Autodesk Inventor part; units mm, degrees
ref_plane "YZ Plane" through (0, 0, 0) normal (1, 0, 0) x (0, 1, 0)
ref_plane "XZ Plane" through (0, 0, 0) normal (0, 1, 0) x (-1, 0, 0)
ref_plane "XY Plane" through (0, 0, 0) normal (0, 0, 1) x (1, 0, 0)
sketch "Sketch1" plane through (0, 0, 0) normal (0, 1, 0) x (-1, 0, 0)
  circle A0 centre (0, 0) radius 4
  dimension "d0" = 8
extrude "Extrusion1" add sketch "Sketch1" along normal blind 36
sketch "Sketch2" plane through (0, 36, 0) normal (0, 1, 0) x (1, 0, 0)
  line L0 (0, -2) -> (2.3553, -2)
  line L1 (-0.9798, -0.8) -> (0.9798, -0.8)
  arc A0 (0.9798, -0.8) -> (-0.9798, -0.8) centre (0, -0.3) ccw
  circle A1 centre (0, 0) radius 4
  line L2 (5.6, 0) -> (-5.6, 0)
  dimension "d4" = 1.2
  dimension "d6" = 1.1
  dimension "d7" = 0.3
extrude "Extrusion2" add sketch "Sketch2" along normal blind 11.25 contours A0 L2 L1 | A0 L2
sketch "Sketch3" plane through (0, 0, 0) normal (0, -1, 0) x (1, 0, 0)
  line L0 (-0.9798, 0.8) -> (0.9798, 0.8)
  arc A0 (-0.9798, 0.8) -> (0.9798, 0.8) centre (0, 0.3) ccw
  point P0 (0, 0)
  point P1 (0, 0)
  point P2 (0, 0.8)
  dimension "d12" = 1.9596
  dimension "d16" = 1.1
  dimension "d17" = 0.3
extrude "Extrusion3" add sketch "Sketch3" along normal blind 9
sketch "Sketch5" plane through (0, 0, 0) normal (0, -1, 0) x (1, 0, 0)
  circle A0 centre (0, 0) radius 5.5
  dimension "d29" = 11
extrude "Extrusion5" add sketch "Sketch5" against normal blind 2
chamfer "Chamfer3" distance 0.5 angle 45 2 edges at (-5.5, 0, 0) (-5.5, 2, 0)
equation "\"d4\" = d3"
properties part number "axle-skibidi"
Here's how the part is built. I have some questions about the finished solid (model axes, mm). A direction names the side the tool comes from. Round coordinates to 2 decimals unless told otherwise and drop trailing zeros. Write each loop counter-clockwise with the first axis right and the second up, starting at its lowest first coordinate (ties: lowest second). Pieces come first, ordered by that corner, then holes. Notation, with made-up numbers: M 62.25,16 L 84.25,16 A27 ccw 84.25,45 Z; hole C -1.5,26.25 d8. An arc over 180 degrees is marked long. Answer as CSV lines item,"result". Start each with the question number.
1. I need wall thicknesses on probe 1 along X at (y, z) = (1, 0.25); probe 2 along X at (y, z) = (-4.5, 0.25); probe 3 along Y at (x, z) = (0.75, 2). Which ranges of each line are inside material? Lowest first, please.
2. Suppose I cut it at D-D on y = -0.5. Write out the boundary of the cut face in (x, z).
3. On a 3-axis mill with a long thin cutter (end or side, diameter ignored), from which of +Z, -Z, +X, -X, +Y, -Y can I reach the whole of each face in a straight line? I mean faces 1 (the flat face through (0, -4, 0.8)), 2 (the cylindrical face through (0, 41.5, -0.8)), 3 (the flat face through (0, 42, 0.8)), 4 (the flat face through (0, 47.25, 0)), 5 (the cylindrical face through (0, -4.4, -0.8)). Say none if no direction works.
4. I'm going to push flat-ended pins straight in: pin 1 Ø4 at (x, y) = (-2, 23.5) entering from +Z; pin 2 Ø3 at (x, y) = (4, 30) entering from +Z; pin 3 Ø1.6 at (x, y) = (0.5, 44) entering from +Z. Where does each tip first touch, or does it pass through?
5. Suppose I cut it at A-A on x = 0. Write out the boundary of the cut face in (y, z).
6. Suppose I cut it at C-C on z = 0. Write out the boundary of the cut face in (x, y), then the cut area to 3 significant figures.
7. Suppose I cut it at B-B on y = 14.5. Write out the boundary of the cut face in (x, z), then the cut area to 3 significant figures.
Check result:
1,probe 1,"x = -5.49 to 5.49"
1,probe 2,"x = -1.1 to 1.1"
1,probe 3,"y = 0 to 36"
2,outline,"M -0.98,0.8 A1.1 ccw long 0.98,0.8 Z"
3,face 1,"+Z, +X, -X, -Y"
3,face 2,"+Y"
3,face 3,"+Z, +X, -X, +Y"
3,face 4,"+Z, -Z, +X, -X, +Y"
3,face 5,"-Y"
4,pin 1,"stops at z = 4"
4,pin 2,"stops at z = 3.12"
4,pin 3,"stops at z = 0.8"
5,outline,"M -9,-0.8 L 0,-0.8 L 0,-5 L 0.5,-5.5 L 1.5,-5.5 L 2,-5 L 2,-4 L 36,-4 L 36,-0.8 L 47.25,-0.8 L 47.25,0.8 L 36,0.8 L 36,4 L 2,4 L 2,5 L 1.5,5.5 L 0.5,5.5 L 0,5 L 0,0.8 L -9,0.8 Z"
6,outline,"M -5.5,0.5 L -5,0 L -1.06,0 L -1.06,-9 L 1.06,-9 L 1.06,0 L 5,0 L 5.5,0.5 L 5.5,1.5 L 5,2 L 4,2 L 4,36 L 1.06,36 L 1.06,47.25 L -1.06,47.25 L -1.06,36 L -4,36 L -4,2 L -5,2 L -5.5,1.5 Z"
6,area,"336 mm2"
7,outline,"C 0,0 d8"
7,area,"50.3 mm2"
